Design review of the part built by this model. Coordinates are the model's own, in mm. Face numbers are marked on the shaded views. A direction names the side the tool comes from. Coordinates: 2 decimals unless noted, no trailing zeros. Write each loop counter-clockwise with the first axis right and the second up, starting at its lowest first coordinate (ties: lowest second). Pieces come first, ordered by that corner, then holes. Notation, with made-up numbers: (-0.5, -23.75) - (48.5, -23.75) arc R23 cw to (48.5, 9.25) - close; hole circle Ø11 at (89, 61). An arc over 180 degrees is marked (long way). One line per item, written item: value.
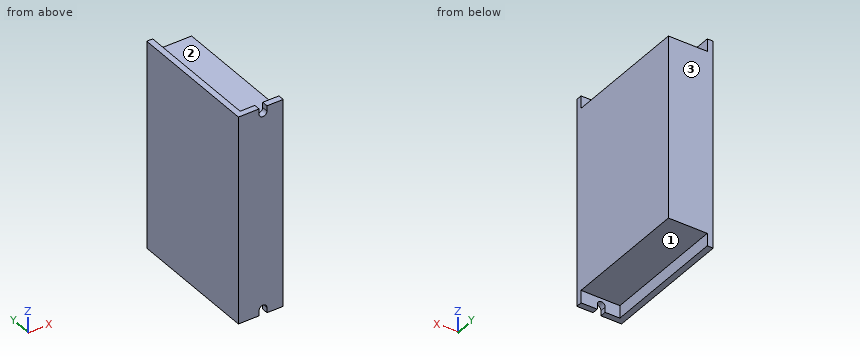
from build123d import *

# Parameters (mm, degrees)
SKETCH2_W           = 25.5
SKETCH2_H           = 118
BOSS_EXTRUDE3_DEPTH = 3.5
CUT_EXTRUDE1_DEPTH  = 4.5
SKETCH4_W           = 3.4
SKETCH4_H           = 118
BOSS_EXTRUDE4_DEPTH = 72
SKETCH5_W           = 22.1
SKETCH5_H           = 103.8
BOSS_EXTRUDE5_DEPTH = 72


with BuildPart() as part:
    # Sketch2 → Boss-Extrude3 (new body)
    with BuildSketch(Plane(origin=(0, 0, 0), x_dir=(1, 0, 0), z_dir=(0, 1, 0))):
        Rectangle(SKETCH2_W, SKETCH2_H)
    extrude(amount=BOSS_EXTRUDE3_DEPTH)

    # Sketch3 → Cut-Extrude1 (cut, through all)
    with BuildSketch(Plane(origin=(0, 3.5, 0), x_dir=(1, 0, 0), z_dir=(0, 1, 0))):
        with BuildLine():
            Line((-1, 56), (-1, 59))
            Line((-1, 59), (3.5, 59))
            Line((3.5, 59), (3.5, 56))
            ThreePointArc((3.5, 56), (1.25, 53.75), (-1, 56))
        make_face()
        with BuildLine():
            Line((-1, -56), (-1, -59))
            Line((-1, -59), (3.5, -59))
            Line((3.5, -59), (3.5, -56))
            ThreePointArc((3.5, -56), (1.25, -53.75), (-1, -56))
        make_face()
    extrude(amount=-CUT_EXTRUDE1_DEPTH, mode=Mode.SUBTRACT)

    # Sketch4 → Boss-Extrude4 (add)
    with BuildSketch(Plane(origin=(0, 3.5, 0), x_dir=(1, 0, 0), z_dir=(0, 1, 0))):
        with Locations((-11.05, 0)):
            Rectangle(SKETCH4_W, SKETCH4_H)
    extrude(amount=BOSS_EXTRUDE4_DEPTH)

    # Sketch5 → Boss-Extrude5 (add)
    with BuildSketch(Plane(origin=(0, 3.5, 0), x_dir=(1, 0, 0), z_dir=(0, 1, 0))):
        with Locations((1.7, 0)):
            Rectangle(SKETCH5_W, SKETCH5_H)
    extrude(amount=BOSS_EXTRUDE5_DEPTH)


solid = part.part
1. Wall thickness on line 1 along Z through (x, y) = (-6.25, 63): over which ranges is the line inside the solid? List them lowest first.
Answer block:
line 1: z = -51.9 to 51.9
2. Consider section B-B, the plane y = 22. Write out the cut boundary in (x, z).
Answer block:
outline: (-12.75, -59) - (-9.35, -59) - (-9.35, -51.9) - (12.75, -51.9) - (12.75, 51.9) - (-9.35, 51.9) - (-9.35, 59) - (-12.75, 59) - close
3. Consider section A-A, the plane x = -3.25. Write out the cut boundary in (y, z).
Answer block:
outline: (0, -59) - (3.5, -59) - (3.5, -51.9) - (75.5, -51.9) - (75.5, 51.9) - (3.5, 51.9) - (3.5, 59) - (0, 59) - close
4. Insertion check: pin 1 Ø5.5 at (y, z) = (54, -56.5) entering from +X; pin 2 Ø12 at (x, y) = (0, 17) entering from -Z; pin 3 Ø3 at (x, y) = (-2, 64.5) entering from +Z. Each pin has a flat end and moves straight along its axis. Give the tip position at first contact, or say it passes through.
Answer block:
pin 1: stops at x = -9.35
pin 2: stops at z = -51.9
pin 3: stops at z = 51.9
5. For the marked faces 1, 2 and 3, list the 3-axis set-ups (+Z, -Z, +X, -X, +Y, -Y) from which the entire face can be reached by the end or side of a thin tool; tool diameter is ignored.
Answer block:
face 1: -Z, +X, +Y
face 2: +Z, +X, +Y
face 3: +Z, -Z, +X, -X, +Y
